Geometry check sheet. Reference: the model listing, model coordinates, mm. A direction names the side the tool comes from. Round coordinates to 2 decimals unless told otherwise and drop trailing zeros. Order: outer loops, then holes, each group sorted by start corner. A loop starts at its lowest first (then second) coordinate and runs counter-clockwise, first axis right, second up.
```python
from build123d import *

# Parameters (mm, degrees)
LEG_DEPTH              = 184
SKETCH5_W              = 20
SKETCH5_H              = 21.25
CELL_SLOTS_DEPTH       = 30
SKETCH6_W              = 20
SKETCH6_H              = 0.25
CELL_SLOTS_TRIM_DEPTH  = 30
SKETCH7_R              = 1.8
SCREW_HOLE_FRONT_DEPTH = 10
SCREW_START            = -10
SKETCH8_R              = 1.8
SCREW_HOLE_BACK_DEPTH  = 10
SKETCH9_W              = 28
SKETCH9_H              = 36
FRONT_TRIM_DEPTH       = 5
SKETCH10_W             = 28
SKETCH10_H             = 36
BACK_TRIM_DEPTH        = 5


with BuildPart() as part:
    # Sketch1 → Leg (new body)
    with BuildSketch(Plane.XY):
        Polygon((0, -6), (0, 0), (0, 30), (-28, 30), (-28, -6), align=None)
    extrude(amount=-LEG_DEPTH)

    # Sketch5 → Cell Slots (cut)
    with BuildSketch(Plane(origin=(0, 30, 0), x_dir=(1, 0, 0), z_dir=(0, 1, 0))):
        with Locations((-10, 33.875)):
            Rectangle(SKETCH5_W, SKETCH5_H)
        with Locations((-10, 10.625)):
            Rectangle(SKETCH5_W, SKETCH5_H)
        with Locations((-10, 57.125)):
            Rectangle(SKETCH5_W, SKETCH5_H)
        with Locations((-10, 80.375)):
            Rectangle(SKETCH5_W, SKETCH5_H)
        with Locations((-10, 103.625)):
            Rectangle(SKETCH5_W, SKETCH5_H)
        with Locations((-10, 126.875)):
            Rectangle(SKETCH5_W, SKETCH5_H)
        with Locations((-10, 150.125)):
            Rectangle(SKETCH5_W, SKETCH5_H)
        with Locations((-10, 173.375)):
            Rectangle(SKETCH5_W, SKETCH5_H)
    extrude(amount=-CELL_SLOTS_DEPTH, mode=Mode.SUBTRACT)

    # Sketch6 → Cell Slots Trim (cut)
    with BuildSketch(Plane(origin=(0, 30, 0), x_dir=(1, 0, 0), z_dir=(0, 1, 0))):
        with Locations((-10, 21.375)):
            Rectangle(SKETCH6_W, SKETCH6_H)
        with Locations((-10, 23.125)):
            Rectangle(SKETCH6_W, SKETCH6_H)
        with Locations((-10, 44.625)):
            Rectangle(SKETCH6_W, SKETCH6_H)
        with Locations((-10, 46.375)):
            Rectangle(SKETCH6_W, SKETCH6_H)
        with Locations((-10, 67.875)):
            Rectangle(SKETCH6_W, SKETCH6_H)
        with Locations((-10, 69.625)):
            Rectangle(SKETCH6_W, SKETCH6_H)
        with Locations((-10, 91.125)):
            Rectangle(SKETCH6_W, SKETCH6_H)
        with Locations((-10, 92.875)):
            Rectangle(SKETCH6_W, SKETCH6_H)
        with Locations((-10, 114.375)):
            Rectangle(SKETCH6_W, SKETCH6_H)
        with Locations((-10, 116.125)):
            Rectangle(SKETCH6_W, SKETCH6_H)
        with Locations((-10, 137.625)):
            Rectangle(SKETCH6_W, SKETCH6_H)
        with Locations((-10, 139.375)):
            Rectangle(SKETCH6_W, SKETCH6_H)
        with Locations((-10, 160.875)):
            Rectangle(SKETCH6_W, SKETCH6_H)
        with Locations((-10, 162.625)):
            Rectangle(SKETCH6_W, SKETCH6_H)
    extrude(amount=-CELL_SLOTS_TRIM_DEPTH, mode=Mode.SUBTRACT)

    # Sketch7 → Screw Hole Front (cut)
    with BuildSketch(Plane.XY):
        with Locations((-24, -3)):
            Circle(SKETCH7_R)
    extrude(amount=-SCREW_HOLE_FRONT_DEPTH, mode=Mode.SUBTRACT)

    # Sketch8 → Screw Hole Back (cut)
    with BuildSketch(Plane(origin=(0, 0, -184), x_dir=(-1, 0, 0), z_dir=(0, 0, -1)).offset(SCREW_START)):
        with Locations(Location((24, -3, 0), (0, 0, 180))):
            Circle(SKETCH8_R)
    extrude(amount=SCREW_HOLE_BACK_DEPTH, mode=Mode.SUBTRACT)

    # Sketch9 → Front Trim (cut)
    with BuildSketch(Plane.XY):
        with Locations((-14, 12)):
            Rectangle(SKETCH9_W, SKETCH9_H)
    extrude(amount=-FRONT_TRIM_DEPTH, mode=Mode.SUBTRACT)

    # Sketch10 → Back Trim (cut)
    with BuildSketch(Plane(origin=(0, 0, -184), x_dir=(-1, 0, 0), z_dir=(0, 0, -1))):
        with Locations((14, 12)):
            Rectangle(SKETCH10_W, SKETCH10_H)
    extrude(amount=-BACK_TRIM_DEPTH, mode=Mode.SUBTRACT)


solid = part.part
```
(1) Sectioned sample at C-C, the plane z = -74.5. Record the cut outline in (x, y), and give its area (3 significant figures).
Returned:
outline: (-28, -6) - (0, -6) - (0, 0) - (-20, 0) - (-20, 30) - (-28, 30) - close
area: 408 mm2
(2) Depth check by flat-ended pin: P1, Ø10, axis at x = -14, y = 22, coming from the +Z side; P2, Ø2, axis at x = -9, z = -30, coming from the +Y side; P3, Ø6, axis at x = -6.5, y = 17.5, coming from the -Z side. Enter the tip coordinate at first touch or a pass-through.
Returned:
P1: stops at z = -21.5
P2: stops at y = 0
P3: stops at z = -162.5
(3) Draft check along Z on faces 5 (the flat face through (-10, 15, -91.25)), 6 (the flat face through (-10, 15, -92.75)), 7 (the flat face through (-24, -3, -174)), 8 (the flat face through (-21, 30, -104)). Enter one of: released by +Z, released by -Z, zero draft, split by the parting line, or undercut.
Returned:
face 5: undercut
face 6: undercut
face 7: released by -Z
face 8: zero draft
(4) Set-up check for faces 1 (the flat face through (-10, 15, -23)), 2 (the cylindrical face through (-22.283, -3.541, -176.465)), 3 (the flat face through (-23, 8, -179)), 4 (the flat face through (-10, 15, -162.5)): record each of +Z, -Z, +X, -X, +Y, -Y from which the full face is reachable in a straight line by a thin tool's end or side.
Returned:
face 1: +X, +Y
face 2: -Z
face 3: -Z, +X, -X, +Y, -Y
face 4: -Z, +X, +Y
(5) Material ranges on line 1 (Y direction, x = -24, z = -6.65); line 2 (X direction, y = -3, z = -177); line 3 (X direction, y = 6, z = -33.5), recorded low to high.
Returned:
line 1: y = -6 to -4.8, -1.2 to 30
line 2: x = -28 to -25.8, -22.2 to 0
line 3: x = -28 to -20
